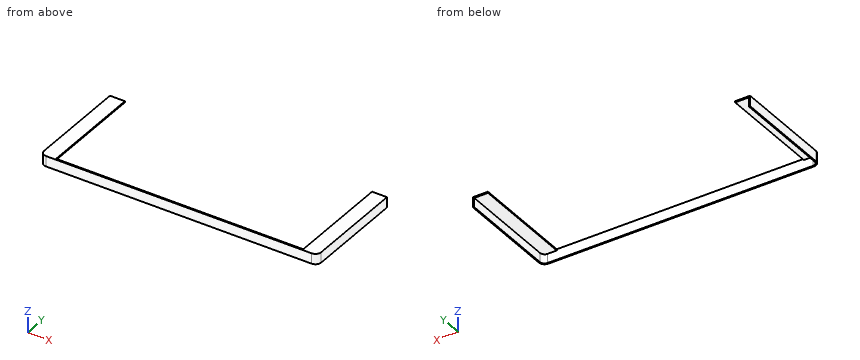
```python
from build123d import *

# Parameters (mm, degrees)
SIDE_DEPTH     = 25.4
PANEL_DEPTH    = 3.4163
BACK_CUT_REACH = 5.416
SKETCH4_W      = 685.8
SKETCH4_H      = 288.6837


with BuildPart() as part:
    # Sketch2 → Side (new body)
    with BuildSketch(Plane.XY):
        with BuildLine():
            Line((-381, 12.7), (-381, 288.6837))
            Line((-381, 288.6837), (-384.4163, 288.6837))
            Line((-384.4163, 288.6837), (-384.4163, 12.7))
            ThreePointArc((-384.4163, 12.7), (-379.695945018, 1.304054982), (-368.3, -3.4163))
            Line((-368.3, -3.4163), (368.3, -3.4163))
            ThreePointArc((368.3, -3.4163), (379.695945018, 1.304054982), (384.4163, 12.7))
            Line((384.4163, 12.7), (384.4163, 288.6837))
            Line((384.4163, 288.6837), (381, 288.6837))
            Line((381, 288.6837), (381, 12.7))
            ThreePointArc((381, 12.7), (377.280256121, 3.719743879), (368.3, 0))
            Line((368.3, 0), (-368.3, 0))
            ThreePointArc((-368.3, 0), (-377.280256121, 3.719743879), (-381, 12.7))
        make_face()
    extrude(amount=-SIDE_DEPTH)

    # Sketch3 → Panel (add)
    with BuildSketch(Plane.XY):
        with BuildLine():
            Line((-368.3, -3.4163), (368.3, -3.4163))
            ThreePointArc((368.3, -3.4163), (379.695945018, 1.304054982), (384.4163, 12.7))
            Line((384.4163, 12.7), (384.4163, 288.6837))
            Line((384.4163, 288.6837), (-384.4163, 288.6837))
            Line((-384.4163, 288.6837), (-384.4163, 12.7))
            ThreePointArc((-384.4163, 12.7), (-379.695945018, 1.304054982), (-368.3, -3.4163))
        make_face()
    extrude(amount=PANEL_DEPTH)

    # Sketch4 → Back Cut (cut, up to next)
    with BuildSketch(Plane(origin=(0, 0, 0), x_dir=(-1, 0, 0), z_dir=(0, 0, -1)), mode=Mode.PRIVATE) as back_cut_sk1:
        with Locations((0, 144.34185)):
            Rectangle(SKETCH4_W, SKETCH4_H)
    back_cut_tool1 = extrude(back_cut_sk1.sketch, amount=-BACK_CUT_REACH, mode=Mode.PRIVATE) & part.part
    add(back_cut_tool1.solids().sort_by_distance((0, 144.34185, 0))[0], mode=Mode.SUBTRACT)


solid = part.part
```
Geometry: final body of the model. Coordinates: model frame, mm. Round coordinates to 2 decimals unless told otherwise and drop trailing zeros. Order: outer loops, then holes, each group sorted by start corner. A loop starts at its lowest first (then second) coordinate and runs counter-clockwise, first axis right, second up. Notation, with made-up numbers: (83, 79.25) -> (134, 79.25) arc R11 cw to (134, 99.25) -> close; hole circle Ø1 at (-2, 10). An arc over 180 degrees is marked (long way). Use one line per item in the form item = value.
(1) Ray query, probe 1 along X at (y, z) = (44, 0.25); probe 2 along X at (y, z) = (22, -1.5); probe 3 along Y at (x, z) = (-36, -6.5). Return the intervals inside material, ascending. Write a range as [from, to].
Results list:
probe_1 = [-384.42, -342.9], [342.9, 384.42]
probe_2 = [-384.42, -381], [381, 384.42]
probe_3 = [-3.42, 0]
(2) First-contact query: pin 1 Ø19 at (x, y) = (-354, 106.5) entering from -Z. Flat tip, straight axial feed; report the tip coordinate or a pass-through.
Results list:
pin_1 = 0
(3) Section C-C on x = -208. Return loops of the section in (y, z).
Results list:
outline = (-3.42, -25.4) -> (0, -25.4) -> (0, 3.42) -> (-3.42, 3.42) -> close
(4) Section B-B on z = -12.5. Return loops of the section in (x, y), and give its area (3 significant figures).
Results list:
outline = (-384.42, 12.7) arc R16.12 ccw to (-368.3, -3.42) -> (368.3, -3.42) arc R16.12 ccw to (384.42, 12.7) -> (384.42, 288.68) -> (381, 288.68) -> (381, 12.7) arc R12.7 cw to (368.3, 0) -> (-368.3, 0) arc R12.7 cw to (-381, 12.7) -> (-381, 288.68) -> (-384.42, 288.68) -> close
area = 4,560 mm^2
(5) Section A-A on y = 240. Return loops of the section in (x, z).
Results list:
outline = (-384.42, -25.4) -> (-381, -25.4) -> (-381, 0) -> (-342.9, 0) -> (-342.9, 3.42) -> (-384.42, 3.42) -> close; (342.9, 0) -> (381, 0) -> (381, -25.4) -> (384.42, -25.4) -> (384.42, 3.42) -> (342.9, 3.42) -> close
